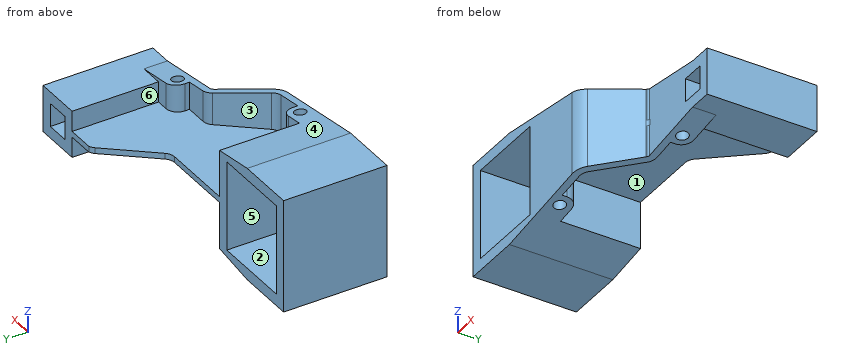
from build123d import *

# Parameters (mm, degrees)
BOSS_EXTRU_3_DEPTH       = 88
ESQUISSE4_W              = 68
ESQUISSE4_H              = 76.5
ENL_V_MAT_EXTRU_1_DEPTH  = 236.459258684
ENL_V_MAT_EXTRU_2_DEPTH  = 68
ENL_V_MAT_EXTRU_5_REACH  = 245.615
ESQUISSE6_W              = 150.690647389
ESQUISSE6_H              = 20
BOSS_EXTRU_5_DEPTH       = 20
ESQUISSE14_W             = 40
ESQUISSE14_H             = 40
ENL_V_MAT_EXTRU_6_DEPTH  = 236.459258684
BOSS_EXTRU_8_DEPTH       = 40
ENL_V_MAT_EXTRU_7_DEPTH  = 236.984242059
ESQUISSE27_W             = 169
ESQUISSE27_H             = 5
BOSS_EXTRU_9_DEPTH       = 45.5
BOSS_EXTRU_10_REACH      = 258.45
ESQUISSE28_R             = 5
ENL_V_MAT_EXTRU_9_DEPTH  = 45.5
BOSS_EXTRU_12_DEPTH      = 17.5
ENL_V_MAT_EXTRU_10_REACH = 248.129
BOSS_EXTRU_13_REACH      = 258.45
ESQUISSE34_R             = 5
BOSS_EXTRU_14_DEPTH      = 17.5
ESQUISSE36_W             = 20
ESQUISSE36_H             = 20
ENL_V_MAT_EXTRU_11_DEPTH = 256.967405152
ESQUISSE37_R             = 5
ENL_V_MAT_EXTRU_12_DEPTH = 10
ESQUISSE38_R             = 5
ENL_V_MAT_EXTRU_13_DEPTH = 10


with BuildPart() as part:
    # Esquisse1 → Boss.-Extru.3 (new body)
    with BuildSketch(Plane(origin=(0, 0, 0), x_dir=(1, 0, 0), z_dir=(0, 1, 0))):
        Polygon((193, 20), (6, 48.25), (-44, 48.25), (-44, -48.25), (6, -48.25), (193, -20), (213, -20), (213, 20), align=None)
    extrude(amount=BOSS_EXTRU_3_DEPTH)

    # Esquisse4 → Enlèv. mat.-Extru.1 (cut, through all)
    with BuildSketch(Plane(origin=(0, 88, 0), x_dir=(1, 0, 0), z_dir=(0, 1, 0))):
        Rectangle(ESQUISSE4_W, ESQUISSE4_H)
    extrude(amount=-ENL_V_MAT_EXTRU_1_DEPTH, mode=Mode.SUBTRACT)

    # Esquisse5 → Enlèv. mat.-Extru.2 (cut)
    with BuildSketch(Plane(origin=(0, 88, 0), x_dir=(1, 0, 0), z_dir=(0, 1, 0))):
        Polygon((193, 20), (173, 20), (173, 2.5), (44, 2.5), (44, 42.509358289), align=None)
        Polygon((173, -20), (193, -20), (44, -42.509358289), (44, -2.5), (173, -2.5), align=None)
    extrude(amount=-ENL_V_MAT_EXTRU_2_DEPTH, mode=Mode.SUBTRACT)

    # Enlèv. mat.-Extru.5: up to this plane
    enl_v_mat_extru_5_end = Plane(origin=(173, 20, 2.5), z_dir=(0, 0, -1))
    # Esquisse6 → Enlèv. mat.-Extru.5 (cut, up to the surface)
    with BuildSketch(Plane(origin=(7.260340781, 0, 48.059600925), x_dir=(0.9887806747234926, 0, -0.14937462064673088), z_dir=(0.14937462064673088, 0, 0.9887806747234927)), mode=Mode.PRIVATE) as enl_v_mat_extru_5_sk1:
        with Locations((112.501854115, 10)):
            Rectangle(ESQUISSE6_W, ESQUISSE6_H)
    enl_v_mat_extru_5_tool1 = split(extrude(enl_v_mat_extru_5_sk1.sketch, amount=-ENL_V_MAT_EXTRU_5_REACH, mode=Mode.PRIVATE), bisect_by=enl_v_mat_extru_5_end, keep=Keep.BOTH, mode=Mode.PRIVATE)
    add(enl_v_mat_extru_5_tool1.solids().sort_by_distance((118.5, 10, 31.254679))[0], mode=Mode.SUBTRACT)

    # Esquisse11 → Boss.-Extru.5 (add)
    with BuildSketch(Plane.XZ.offset(-20)):
        Polygon((37.955805499, 2.5), (44, 2.5), (44, 42.509358289), align=None)
    extrude(amount=BOSS_EXTRU_5_DEPTH)

    # Esquisse14 → Enlèv. mat.-Extru.6 (cut, through all)
    with BuildSketch(Plane(origin=(0, 88, 0), x_dir=(1, 0, 0), z_dir=(0, 1, 0))):
        with Locations((193, 0)):
            Rectangle(ESQUISSE14_W, ESQUISSE14_H)
    extrude(amount=-ENL_V_MAT_EXTRU_6_DEPTH, mode=Mode.SUBTRACT)

    # Esquisse22 → Boss.-Extru.8 (add)
    with BuildSketch(Plane(origin=(173, 0, 0), x_dir=(0, 0, -1), z_dir=(1, 0, 0))):
        Polygon((-2.5, 0), (20, 0), (20, 20), (2.5, 20), (2.5, 88), (-2.5, 88), align=None)
    extrude(amount=BOSS_EXTRU_8_DEPTH)

    # Esquisse23 → Enlèv. mat.-Extru.7 (cut, through all)
    with BuildSketch(Plane.XY.offset(2.5)):
        with BuildLine():
            Line((213, 0), (213, 40))
            Line((213, 40), (193, 40))
            Line((193, 40), (159, 40))
            Line((159, 40), (134.690473047, 40))
            ThreePointArc((134.690473047, 40), (133, 39.625231148), (131.626295274, 38.571150439))
            Line((131.626295274, 38.571150439), (104.057045727, 5.715398245))
            ThreePointArc((104.057045727, 5.715398245), (98.562226825, 1.499075407), (91.800334637, 0))
            Line((91.800334637, 0), (213, 0))
        make_face()
    extrude(amount=-ENL_V_MAT_EXTRU_7_DEPTH, mode=Mode.SUBTRACT)

    # Esquisse27 → Boss.-Extru.9 (add)
    with BuildSketch(Plane(origin=(0, 88, 0), x_dir=(1, 0, 0), z_dir=(0, 1, 0))):
        with Locations((128.5, 0)):
            Rectangle(ESQUISSE27_W, ESQUISSE27_H)
    extrude(amount=BOSS_EXTRU_9_DEPTH)

    # Boss.-Extru.10: up to this plane
    boss_extru_10_end = Plane(origin=(7.260340781, 88, 48.059600925), z_dir=(-0.14937462064673085, 0, -0.9887806747234926))
    # Esquisse28 → Boss.-Extru.10 (add, up to the surface)
    with BuildSketch(Plane.XY.offset(2.5), mode=Mode.PRIVATE) as boss_extru_10_sk1:
        with BuildLine():
            Line((132.074257782, 39.025792076), (132.14881397, 39.114644681))
            ThreePointArc((132.14881397, 39.114644681), (133, 39.767782693), (134.047464579, 40))
            Line((134.047464579, 40), (134.690473047, 40))
            Line((134.690473047, 40), (159, 40))
            Line((159, 40), (193, 40))
            Line((193, 40), (193, 60))
            Line((193, 60), (173, 60))
            Line((173, 60), (163, 60))
            ThreePointArc((163, 60), (155.928932188, 57.071067812), (153, 50))
            Line((153, 50), (153, 46))
            Line((153, 46), (134.690473047, 46))
            ThreePointArc((134.690473047, 46), (130.46429043, 45.06307787), (127.030028616, 42.427876097))
            Line((127.030028616, 42.427876097), (99.460779068, 9.572123903))
            ThreePointArc((99.460779068, 9.572123903), (96.026517254, 6.93692213), (91.800334637, 6))
            Line((91.800334637, 6), (69, 6))
            Line((69, 6), (69, 10))
            ThreePointArc((69, 10), (66.071067812, 17.071067812), (59, 20))
            Line((59, 20), (44, 20))
            Line((44, 20), (44, 0))
            Line((44, 0), (63, 0))
            Line((63, 0), (91.800334637, 0))
            ThreePointArc((91.800334637, 0), (98.562226825, 1.499075407), (104.057045727, 5.715398245))
            Line((104.057045727, 5.715398245), (131.626295274, 38.571150439))
            ThreePointArc((131.626295274, 38.571150439), (131.841194012, 38.807420343), (132.074257782, 39.025792076))
        make_face()
        with Locations((59, 10)):
            Circle(ESQUISSE28_R, mode=Mode.SUBTRACT)
        with Locations((163, 50)):
            Circle(ESQUISSE28_R, mode=Mode.SUBTRACT)
    boss_extru_10_tool1 = split(extrude(boss_extru_10_sk1.sketch, amount=BOSS_EXTRU_10_REACH, mode=Mode.PRIVATE), bisect_by=boss_extru_10_end, keep=Keep.BOTH, mode=Mode.PRIVATE)
    add(boss_extru_10_tool1.solids().sort_by_distance((124.318782, 30.344637, 2.5))[0])

    # Esquisse29 → Enlèv. mat.-Extru.9 (cut)
    with BuildSketch(Plane.XY.offset(2.5)):
        with BuildLine():
            ThreePointArc((145.939599002, 130.613536933), (147.768845256, 132.309522469), (149.96093833, 133.5))
            Line((149.96093833, 133.5), (44, 133.5))
            Line((44, 133.5), (44, 88))
            Line((44, 88), (105.519519296, 88))
            ThreePointArc((105.519519296, 88), (109.745701914, 88.93692213), (113.179963727, 91.572123903))
            Line((113.179963727, 91.572123903), (145.939599002, 130.613536933))
        make_face()
    extrude(amount=-ENL_V_MAT_EXTRU_9_DEPTH, mode=Mode.SUBTRACT)

    # Esquisse31 → Boss.-Extru.12 (add)
    with BuildSketch(Plane.XY.offset(2.5)):
        Polygon((213, 133.5), (173, 133.5), (173, 60), (193, 60), (193, 40), (213, 40), align=None)
    extrude(amount=BOSS_EXTRU_12_DEPTH)

    # Esquisse33 → Enlèv. mat.-Extru.10 (cut, up to next)
    with BuildSketch(Plane(origin=(0, 20, 0), x_dir=(1, 0, 0), z_dir=(0, 1, 0)), mode=Mode.PRIVATE) as enl_v_mat_extru_10_sk1:
        Polygon((44, 42.509358289), (44, 2.5), (116.043249791, 2.5), (116.043249791, 31.625819216), align=None)
    enl_v_mat_extru_10_tool1 = extrude(enl_v_mat_extru_10_sk1.sketch, amount=-ENL_V_MAT_EXTRU_10_REACH, mode=Mode.PRIVATE) & part.part
    add(enl_v_mat_extru_10_tool1.solids().sort_by_distance((78.131402, 20, -19.926572))[0], mode=Mode.SUBTRACT)

    # Boss.-Extru.13: up to this plane
    boss_extru_13_end = Plane(origin=(7.260340781, 88, -48.059600925), z_dir=(0.14937462064673085, 0, -0.9887806747234926))
    # Esquisse34 → Boss.-Extru.13 (add, up to the surface)
    with BuildSketch(Plane(origin=(0, 0, -2.5), x_dir=(-1, 0, 0), z_dir=(0, 0, -1)), mode=Mode.PRIVATE) as boss_extru_13_sk1:
        with BuildLine():
            Line((-44, 0), (-44, 20))
            Line((-44, 20), (-59, 20))
            ThreePointArc((-59, 20), (-66.071067812, 17.071067812), (-69, 10))
            Line((-69, 10), (-69, 6))
            Line((-69, 6), (-91.800334637, 6))
            ThreePointArc((-91.800334637, 6), (-96.026517254, 6.93692213), (-99.460779068, 9.572123903))
            Line((-99.460779068, 9.572123903), (-127.030028616, 42.427876097))
            ThreePointArc((-127.030028616, 42.427876097), (-130.46429043, 45.06307787), (-134.690473047, 46))
            Line((-134.690473047, 46), (-153, 46))
            Line((-153, 46), (-153, 50))
            ThreePointArc((-153, 50), (-155.928932188, 57.071067812), (-163, 60))
            Line((-163, 60), (-173, 60))
            Line((-173, 60), (-193, 60))
            Line((-193, 60), (-193, 40))
            Line((-193, 40), (-159, 40))
            Line((-159, 40), (-134.690473047, 40))
            Line((-134.690473047, 40), (-134.047464579, 40))
            ThreePointArc((-134.047464579, 40), (-133, 39.767782693), (-132.14881397, 39.114644681))
            Line((-132.14881397, 39.114644681), (-132.074257782, 39.025792076))
            ThreePointArc((-132.074257782, 39.025792076), (-131.841194012, 38.807420343), (-131.626295274, 38.571150439))
            Line((-131.626295274, 38.571150439), (-104.057045727, 5.715398245))
            ThreePointArc((-104.057045727, 5.715398245), (-98.562226825, 1.499075407), (-91.800334637, 0))
            Line((-91.800334637, 0), (-63, 0))
            Line((-63, 0), (-44, 0))
        make_face()
        with Locations(Location((-163, 50, 0), (0, 0, 180))):
            Circle(ESQUISSE34_R, mode=Mode.SUBTRACT)
        with Locations(Location((-59, 10, 0), (0, 0, 180))):
            Circle(ESQUISSE34_R, mode=Mode.SUBTRACT)
    boss_extru_13_tool1 = split(extrude(boss_extru_13_sk1.sketch, amount=BOSS_EXTRU_13_REACH, mode=Mode.PRIVATE), bisect_by=boss_extru_13_end, keep=Keep.BOTH, mode=Mode.PRIVATE)
    add(boss_extru_13_tool1.solids().sort_by_distance((124.318782, 30.344637, -2.5))[0])

    # Esquisse35 → Boss.-Extru.14 (add)
    with BuildSketch(Plane(origin=(0, 0, -2.5), x_dir=(-1, 0, 0), z_dir=(0, 0, -1))):
        Polygon((-173, 60), (-173, 133.5), (-213, 133.5), (-213, 40), (-193, 40), (-193, 60), align=None)
    extrude(amount=BOSS_EXTRU_14_DEPTH)

    # Esquisse36 → Enlèv. mat.-Extru.11 (cut, through all)
    with BuildSketch(Plane(origin=(0, 133.5, 0), x_dir=(1, 0, 0), z_dir=(0, 1, 0))):
        with Locations((193, 0)):
            Rectangle(ESQUISSE36_W, ESQUISSE36_H)
    extrude(amount=-ENL_V_MAT_EXTRU_11_DEPTH, mode=Mode.SUBTRACT)

    # Esquisse37 → Enlèv. mat.-Extru.12 (cut)
    with BuildSketch(Plane.XY.offset(2.5)):
        with Locations((59, 10)):
            Circle(ESQUISSE37_R)
    extrude(amount=-ENL_V_MAT_EXTRU_12_DEPTH, mode=Mode.SUBTRACT)

    # Esquisse38 → Enlèv. mat.-Extru.13 (cut)
    with BuildSketch(Plane.XY.offset(2.5)):
        with Locations((163, 50)):
            Circle(ESQUISSE38_R)
    extrude(amount=-ENL_V_MAT_EXTRU_13_DEPTH, mode=Mode.SUBTRACT)


solid = part.part
Can you work these out from the model? Positions are in its coordinate system, mm. Face numbers are marked on the shaded views. A direction names the side the tool comes from. Give positions to 0.01 mm unless a question says otherwise; leave off trailing zeros. Order: outer loops, then holes, each group sorted by start corner. A loop starts at its lowest first (then second) coordinate and runs counter-clockwise, first axis right, second up. Notation, with made-up numbers: M 1,3 L 49,3 A9 ccw 49,7 Z; hole C 89,60 d2. An arc over 180 degrees is marked long. One line per question, with ' | ' between items.
Item 1: Suppose I cut it at B-B, the plane y = 26. Write out the boundary of the cut face in (x, z).
Answer block:
outline: M -44,-48.25 L 6,-48.25 L 44,-42.51 L 44,-2.5 L 113.25,-2.5 L 113.25,-32.05 L 121.08,-30.87 L 121.08,30.87 L 113.25,32.05 L 113.25,2.5 L 44,2.5 L 44,42.51 L 6,48.25 L -44,48.25 Z; hole M -34,-38.25 L 34,-38.25 L 34,38.25 L -34,38.25 Z
Item 2: For the marked faces 1, 2 and 3, which set-ups out of +Z, -Z, +X, -X, +Y, -Y let a thin tool reach every point of the face, with its end or its side?
Answer block:
face 1: -Z, +Y | face 2: +Y, -Y | face 3: +Z, +Y
Item 3: Please list where these lines run through material, in increasing order: L1, parallel to X at y = 50, z = 2; L2, parallel to X at y = 50, z = 7; L3, parallel to X at y = 79, z = 13.
Answer block:
L1: x = -44 to -34, 34 to 158, 168 to 183, 203 to 213 | L2: x = -44 to -34, 34 to 44, 153 to 158, 168 to 183, 203 to 213 | L3: x = -44 to -34, 34 to 44, 173 to 213
Item 4: Suppose I cut it at A-A, the plane x = -25. Write out the boundary of the cut face in (y, z), then the cut area to 3 significant figures.
Answer block:
outline: M 0,-48.25 L 88,-48.25 L 88,-38.25 L 0,-38.25 Z; M 0,38.25 L 88,38.25 L 88,48.25 L 0,48.25 Z | area: 1,760 mm2
Item 5: We'd pull the mould along Z, two halves only. Please class the marked faces 4, 5 and 6: released by +Z, released by -Z, zero draft, split by the parting line, or undercut.
Answer block:
face 4: released by +Z | face 5: undercut | face 6: zero draft
Item 6: I'm going to push flat-ended pins straight in: pin 1 Ø25 at (x, z) = (80, 24) entering from +Y; pin 2 Ø12 at (x, z) = (53.5, 20.5) entering from +Y; pin 3 Ø18 at (x, z) = (76, -26) entering from +Y. Where does each tip first touch, or does it pass through?
Answer block:
pin 1: stops at y = 15.27 | pin 2: stops at y = 20 | pin 3: stops at y = 16
Item 7: Suppose I cut it at C-C, the plane y = 97. Write out the boundary of the cut face in (x, z).
Answer block:
outline: M 117.73,-2.5 L 173,-2.5 L 173,-20 L 213,-20 L 213,20 L 173,20 L 173,2.5 L 117.73,2.5 Z; hole M 183,-10 L 203,-10 L 203,10 L 183,10 Z
